Model file for the job. Use its own axes, mm. A direction names the side the tool comes from. Round coordinates to 2 decimals unless told otherwise and drop trailing zeros. Write each loop counter-clockwise with the first axis right and the second up, starting at its lowest first coordinate (ties: lowest second). Pieces come first, ordered by that corner, then holes. Notation, with made-up numbers: (45, -15) - (55, -15) arc R21 cw to (55, -9) - close; hole circle Ø11 at (76, 9.5). An arc over 180 degrees is marked (long way). One line per item, written item: value.
Solid Edge part; units mm, degrees
sketch "Sketch1" plane through (0, 0, 0) normal (0, 0, 1) x (1, 0, 0)
  circle A0 centre (0, 0) radius 20
extrude "Protrusion1" add sketch "Sketch1" against normal blind 35
sketch "Sketch2" plane through (0, 0, 0) normal (1, 0, 0) x (0, 1, 0)
  line L0 (-40, 0) -> (-100, -65)
  line L1 (-100, -65) -> (0, -65)
  line L2 (0, -65) -> (0, 0)
  line L3 (0, 0) -> (-40, 0)
extrude "拉延_2" add sketch "Sketch2" along normal mid plane 15
sketch "Sketch3" plane through (0, 0, 0) normal (1, 0, 0) x (0, 1, 0)
  line L0 (-40, -80) -> (-40, -65)
  line L1 (-40, -65) -> (-100, -65)
  line L2 (-100, -65) -> (-100, -80)
  line L3 (-100, -80) -> (-40, -80)
extrude "拉延_3" add sketch "Sketch3" along normal mid plane 80
sketch "Sketch4" plane through (40, 0, 0) normal (1, 0, 0) x (0, 1, 0)
  line L0 (-18.5405, -30) -> (29.7908, -30)
  line L1 (29.7908, -65) -> (29.7908, -30)
  line L2 (-40, -65) -> (29.7908, -65)
  line L3 (-18.5405, -30) -> (-40, -65)
extrude "Cutout1" cut sketch "Sketch4" against normal up to next
sketch "Sketch5" plane through (0, -10, 0) normal (0, 0, 1) x (0, 1, 0)
  circle A0 centre (10, 0) radius 10
extrude "Cutout2" cut sketch "Sketch5" against normal up to next
sketch "Sketch6" plane through (23.75, -70, -65) normal (0, 0, 1) x (0, 1, 0)
  circle A0 centre (13.0142, -2.0485) radius 5
  circle A1 centre (-11.4477, -0.6025) radius 5
extrude "Cutout3" cut sketch "Sketch6" against normal up to next
properties material "ABS Plastic, high impact"
1. Mould opens along X. For faces 4 (the face through (7.5, -51, -40)), 5 (the face through (0.772, 19.985, -14.79)), 6 (the face through (26.27, -76.83, -72.4)), 7 (the face through (0.105, -29.12, -47.255)) say: released by +X, released by -X, zero draft, split by the parting line, or undercut.
Report:
face 4: released by +X
face 5: split by the parting line
face 6: undercut
face 7: zero draft
2. Band-saw the part on C-C on y = -46. Write the cut outline in (x, z), plus the area to 3 significant figures.
Report:
outline: (-40, -80) - (40, -80) - (40, -65) - (7.5, -65) - (7.5, -6.5) - (-7.5, -6.5) - (-7.5, -65) - (-40, -65) - close
area: 2,080 mm²
3. Drop flat-ended pins along their axis: pin 1 (3 mm diameter, centred on x = 0.5, z = -36.5, fed in from +Y); pin 2 (1.5 mm diameter, centred on x = -11, z = -16, fed in from -Y); pin 3 (10 mm diameter, centred on x = -28.5, y = -82.5, fed in from +Z). Give the stop position or say it passes through.
Report:
pin 1: y = -21.61
pin 2: y = -17.17
pin 3: z = -65
4. Band-saw the part on D-D on z = -14. Write the cut outline in (x, y).
Report:
outline: (-7.5, -52.92) - (7.5, -52.92) - (7.5, -18.54) arc R20 ccw (long way) to (-7.5, -18.54) - close; hole circle Ø20 at (0, 0)
5. Tool access for faces 1 (the face through (24, -70, -65)), 2 (the face through (5, 9, -30)), 3 (the face through (-24, -70, -65)): list every direction of +Z, -Z, +X, -X, +Y, -Y with a clear straight run to the whole face (end or side of a thin tool).
Report:
face 1: +Z, +X, +Y, -Y
face 2: -Z, +X, -X, +Y
face 3: +Z, -X, +Y, -Y
6. Band-saw the part on A-A on x = 0. Write the cut outline in (y, z), plus the area to 3 significant figures.
Report:
outline: (-100, -80) - (-40, -80) - (-40, -65) - (-18.54, -30) - (-10, -30) - (-10, 0) - (-40, 0) - (-100, -65) - close; (10, -30) - (20, -30) - (20, 0) - (10, 0) - close
area: 4,430 mm²
7. Band-saw the part on B-B on y = 0. Write the cut outline in (x, z).
Report:
outline: (-20, -30) - (-10, -30) - (-10, 0) - (-20, 0) - close; (10, -30) - (20, -30) - (20, 0) - (10, 0) - close
8. Wall check: probe 1 along X at (y, z) = (0, -13.5); probe 2 along X at (y, z) = (-57.5, -31.5); probe 3 along Y at (x, z) = (0, -15). Give the ranges that are in metal, low to high. Write a range as [from, to].
Report:
probe 1: [-20, -10], [10, 20]
probe 2: [-7.5, 7.5]
probe 3: [-53.85, -10], [10, 20]
